Check sheet for the modelled part. Datum: model origin and axes. Units: mm. Round coordinates to 2 decimals unless told otherwise and drop trailing zeros. Write each loop counter-clockwise with the first axis right and the second up, starting at its lowest first coordinate (ties: lowest second). Pieces come first, ordered by that corner, then holes. Notation, with made-up numbers: (1, 7.25) -> (55, 7.25) arc R19 ccw to (55, 41.25) -> close; hole circle Ø6 at (33.25, -5.75). An arc over 180 degrees is marked (long way). One line per item, written item: value.
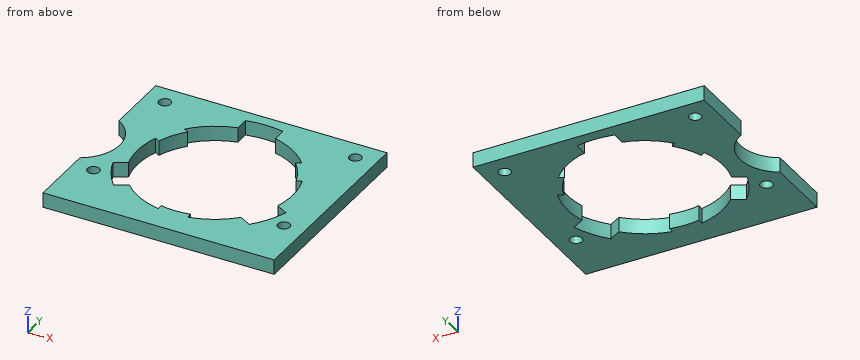
from build123d import *

# Parameters (mm, degrees)
SKETCH1_W             = 43.18
SKETCH1_H             = 38.1
BOSS_EXTRUDE1_DEPTH   = 2.7686
SKETCH2_R             = 14.5
CUT_EXTRUDE1_DEPTH    = 29.925693526
CUT_EXTRUDE2_DEPTH    = 29.925693526
CIRPATTERN1_COUNT     = 3
BOSS_EXTRUDE2_DEPTH   = 2.7686
CIRPATTERN2_COUNT     = 3
SKETCH6_R             = 7.62
CUT_EXTRUDE4_DEPTH    = 29.925693526
F_4_40_TAPPED_HOLE1_D = 2.2606


with BuildPart() as part:
    # Sketch1 → Boss-Extrude1 (new body)
    with BuildSketch(Plane.XY):
        Rectangle(SKETCH1_W, SKETCH1_H)
    extrude(amount=BOSS_EXTRUDE1_DEPTH)

    # Sketch2 → Cut-Extrude1 (cut, through all)
    with BuildSketch(Plane.XY.offset(2.7686)):
        Circle(SKETCH2_R)
    extrude(amount=-CUT_EXTRUDE1_DEPTH, mode=Mode.SUBTRACT)

    # Sketch3 → Cut-Extrude2 (cut, through all)
    with BuildSketch(Plane.XY.offset(2.7686)):
        with BuildLine():
            Line((-3.5, 16.63580476), (-3.5, 14.071247279))
            ThreePointArc((-3.5, 14.071247279), (0, 14.5), (3.5, 14.071247279))
            Line((3.5, 14.071247279), (3.5, 16.63580476))
            ThreePointArc((3.5, 16.63580476), (0, 17), (-3.5, 16.63580476))
        make_face()
    cut_extrude2 = extrude(amount=-CUT_EXTRUDE2_DEPTH, mode=Mode.SUBTRACT)

    # CirPattern1: Cut-Extrude2 ×3 about axis
    cirpattern1_axis = Axis((0, 0, 0), (0, 0, 1))
    for i in range(1, CIRPATTERN1_COUNT):
        add(cut_extrude2.rotate(cirpattern1_axis, i * 360 / CIRPATTERN1_COUNT), mode=Mode.SUBTRACT)

    # Sketch4 → Boss-Extrude2 (add)
    with BuildSketch(Plane.XY.offset(2.7686)):
        with BuildLine():
            Line((-2.75, -13.216939888), (-2.75, -14.236836025))
            ThreePointArc((-2.75, -14.236836025), (0, -14.5), (2.75, -14.236836025))
            Line((2.75, -14.236836025), (2.75, -13.216939888))
            ThreePointArc((2.75, -13.216939888), (0, -13.5), (-2.75, -13.216939888))
        make_face()
    boss_extrude2 = extrude(amount=-BOSS_EXTRUDE2_DEPTH)

    # CirPattern2: Boss-Extrude2 ×3 about axis
    cirpattern2_axis = Axis((0, 0, 0), (0, 0, 1))
    for i in range(1, CIRPATTERN2_COUNT):
        add(boss_extrude2.rotate(cirpattern2_axis, i * 360 / CIRPATTERN2_COUNT))

    # Sketch6 → Cut-Extrude4 (cut, through all)
    with BuildSketch(Plane.XY.offset(2.7686)):
        with Locations((-25.4, 0)):
            Circle(SKETCH6_R)
    extrude(amount=-CUT_EXTRUDE4_DEPTH, mode=Mode.SUBTRACT)

    # #4-40 Tapped Hole1 (through all)
    with Locations(Plane(origin=(0, 0, 0), x_dir=(-1, 0, 0), z_dir=(0, 0, -1))):
        with Locations((-17.78, 15.24), (-17.78, -8.89), (17.78, -8.89), (17.78, 15.24)):
            Hole(F_4_40_TAPPED_HOLE1_D / 2)


solid = part.part
Item 1: Sectioned sample at B-B (x = 17.78). Enter the section's corners in (y, z), then the cut area to 3 significant figures.
Result set:
outline: (-19.05, 0) -> (-10.02, 0) -> (-10.02, 2.77) -> (-19.05, 2.77) -> close; (-7.76, 0) -> (14.11, 0) -> (14.11, 2.77) -> (-7.76, 2.77) -> close; (16.37, 0) -> (19.05, 0) -> (19.05, 2.77) -> (16.37, 2.77) -> close
area: 93.0 mm^2
Item 2: Material ranges on line 1 along Y through (x, z) = (17.78, 1.3); line 2 along Y through (x, z) = (-0.5, 0.7); line 3 along X through (y, z) = (15, 1.6), recorded low to high.
Result set:
line 1: -19.05 to -10.02, -7.76 to 14.11, 16.37 to 19.05
line 2: -19.05 to -13.49, 16.99 to 19.05
line 3: -21.59 to -18.88, -16.68 to -3.5, 3.5 to 16.68, 18.88 to 21.59
Item 3: Sectioned sample at C-C (z = 0.5). State how many separate pieces and enclosed holes the cut face has, then the cut area to 3 significant figures.
Result set:
separate pieces: 1
enclosed holes: 5
area: 897 mm^2
Item 4: Depth check by flat-ended pin: pin 1 (2 mm diameter, centred on x = 15, y = -4, fed in from -Z). Enter the tip coordinate at first touch or a pass-through.
Result set:
pin 1: z = 0
Item 5: Sectioned sample at D-D (x = -9). Enter the section's corners in (y, z), then the cut area to 3 significant figures.
Result set:
outline: (-19.05, 0) -> (-11.37, 0) -> (-11.37, 2.77) -> (-19.05, 2.77) -> close; (11.37, 0) -> (19.05, 0) -> (19.05, 2.77) -> (11.37, 2.77) -> close
area: 42.5 mm^2
Item 6: Sectioned sample at A-A (y = 15.24). Enter the section's corners in (x, z), then the cut area to 3 significant figures.
Result set:
outline: (-21.59, 0) -> (-18.91, 0) -> (-18.91, 2.77) -> (-21.59, 2.77) -> close; (-16.65, 0) -> (-3.5, 0) -> (-3.5, 2.77) -> (-16.65, 2.77) -> close; (3.5, 0) -> (16.65, 0) -> (16.65, 2.77) -> (3.5, 2.77) -> close; (18.91, 0) -> (21.59, 0) -> (21.59, 2.77) -> (18.91, 2.77) -> close
area: 87.7 mm^2
